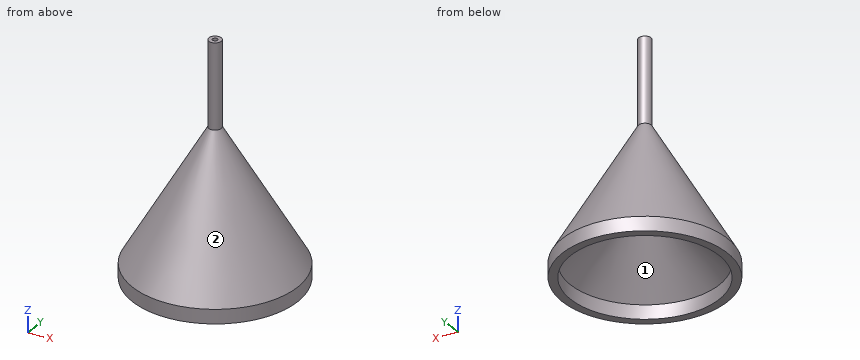
```python
from build123d import *

# Parameters (mm, degrees)
F0_R        = 12.7
F1_DEPTH    = 22.86
F2_R        = 0.9525
F3_DEPTH    = 12.7
F4_R        = 0.381
F5_DEPTH    = 35.561
F6_S5_R     = 0.9525
F6_T6_DEPTH = 22
F7_R        = 11.43
F8_DEPTH    = 1.27
F9_S5_R     = 11.43
F9_T6_DEPTH = 20


# Not quite as in the source:
# - a fillet or chamfer that OpenCascade refuses, or shapes differently, is made with other operations: its cross-section is extruded or revolved along the edge and cut away or added


with BuildPart() as f1:
    # F0 (on Top) → F1 (new body)
    with BuildSketch(Plane.XY):
        with Locations((-32.7860526741, 35.493157804)):
            Circle(F0_R)
    extrude(amount=F1_DEPTH)

    # F2 (on face) → F3 (join)
    with BuildSketch(Plane.XY.offset(22.86)):
        with Locations((-32.7860526741, 35.493157804)):
            Circle(F2_R)
    extrude(amount=F3_DEPTH)

    # F4 (on face) → F5 (cut, through all)
    with BuildSketch(Plane.XY.offset(35.56)):
        with Locations((-32.7860526741, 35.493157804)):
            Circle(F4_R)
    extrude(amount=-F5_DEPTH, mode=Mode.SUBTRACT)

    # F6: chamfer of 11.938 x 20.6772225408 on 1 edges, made by hand


with BuildPart() as f6_tool2:
    # F6_s3 → F6_t4 (revolve)
    with BuildSketch(Plane.XZ.offset(-35.493157804)):
        Polygon((-20.0860526741, 2.1827774592), (-32.0240526741, 22.86), (-20.0860526741, 22.86), align=None)
    revolve(axis=Axis((-32.7860526741, 35.493157804, 22.86), (0, 0, 1)))

    # F6_s5 → F6_t6 (cut, symmetric)
    with BuildSketch(Plane.XY.offset(12.5)):
        with Locations((-32.7860526741, 35.493157804)):
            Circle(F6_S5_R)
    extrude(amount=F6_T6_DEPTH, both=True, mode=Mode.SUBTRACT)


with BuildPart() as f1_1:
    add(f1.part)

    # F6_t1: cut F6_tool2
    add(f6_tool2.part, mode=Mode.SUBTRACT)

    # F7 (on face) → F8 (cut)
    with BuildSketch(Plane(origin=(0, 0, 0), x_dir=(1, 0, 0), z_dir=(0, 0, -1))):
        with Locations((-32.7860526741, -35.493157804)):
            Circle(F7_R)
    extrude(amount=-F8_DEPTH, mode=Mode.SUBTRACT)

    # F9: chamfer of 11.938 on 1 edges, made by hand


with BuildPart() as f9_tool2:
    # F9_s3 → F9_t4 (revolve)
    with BuildSketch(Plane.XZ.offset(-35.493157804)):
        Polygon((-20.4670526741, 1.27), (-32.4050526741, 13.208), (-32.4050526741, 1.27), align=None)
    revolve(axis=Axis((-32.7860526741, 35.493157804, 1.27), (0, 0, 1)))

    # F9_s5 → F9_t6 (intersect, symmetric)
    with BuildSketch(Plane.XY.offset(7.2)):
        with Locations((-32.7860526741, 35.493157804)):
            Circle(F9_S5_R)
    extrude(amount=F9_T6_DEPTH, both=True, mode=Mode.INTERSECT)


with BuildPart() as f1_2:
    add(f1_1.part)

    # F9_t1: cut F9_tool2
    add(f9_tool2.part, mode=Mode.SUBTRACT)


solid = f1_2.part
```
The model under review builds one solid part; all positions refer to its coordinate system, in mm. Face numbers are marked on the shaded views. Give positions to 0.01 mm unless a question says otherwise; leave off trailing zeros. Write each loop counter-clockwise with the first axis right and the second up, starting at its lowest first coordinate (ties: lowest second). Pieces come first, ordered by that corner, then holes. Notation, with made-up numbers: (-33, -25) -> (-27, -25) arc R21 ccw to (-27, -12) -> close; hole circle Ø10 at (66, 87.5). An arc over 180 degrees is marked (long way). Answer in a Markdown table with one row per item.
1) Add section A-A on z = 7.5. State the section outline as (x, y) points.
Worked answers:
| item | result |
|---|---|
| outline | circle Ø19.26 at (-32.79, 35.49); hole circle Ø12.18 at (-32.79, 35.49) |
2) For L1, parallel to X at y = 41.5, z = 6.5; L2, parallel to Y at x = -39.5, z = 3.5; L3, parallel to Y at x = -37.5, z = 3, list the stretches that pass through material, from the lowest coordinate up. Write a range as [from, to].
Worked answers:
| item | result |
|---|---|
| L1 | [-41.04, -36.55], [-29.02, -24.53] |
| L2 | [25.62, 27.96], [43.02, 45.37] |
| L3 | [24.21, 26.01], [44.98, 46.78] |
3) Add section B-B on z = 28. State the section outline as (x, y) points (1 decimal), plus the area to 3 significant figures.
Worked answers:
| item | result |
|---|---|
| outline | circle Ø1.9 at (-32.8, 35.5); hole circle Ø0.8 at (-32.8, 35.5) |
| area | 2.39 mm² |
4) Mouldability with a two-part tool opening along X and no side actions: class the marked faces 1 and 2 as +X half, -X half, draft (parallel to the pull), parting line (faces both ways), or undercut.
Worked answers:
| item | result |
|---|---|
| face 1 | undercut |
| face 2 | parting line |
5) Clearance check with flat-ended pins moving along their axes: P1, Ø2, axis at x = -24, z = 4, coming from the -Y side; P2, Ø3, axis at x = -36, z = 10.5, coming from the -Y side; P3, Ø12, axis at x = -42, y = 32, coming from the +Z side. State where each tip first meets the part, or that it passes through.
Worked answers:
| item | result |
|---|---|
| P1 | y = 26.54 |
| P2 | y = 27.2 |
| P3 | z = 17.5 |
